from build123d import *

# Parameters (mm, degrees)
F1_DEPTH = 14
F2_R     = 5.5
F3_DEPTH = 1
F5_DEPTH = 2


with BuildPart() as f1:
    # F0 (on Top) → F1 (new body)
    with BuildSketch(Plane.XY):
        Polygon((-12.25, 0.3), (-12.25, 9), (-28.25, 9), (-28.25, -9), (12.25, -9), (12.25, 0.3), align=None)
        Polygon((28.25, -9), (28.25, 9), (12.25, 9), (12.25, 0.3), (12.25, -9), align=None)
    extrude(amount=F1_DEPTH)

    # F2 (on face) → F3 (join)
    with BuildSketch(Plane(origin=(0, 9, 0), x_dir=(-1, 0, 0), z_dir=(0, 1, 0))):
        with Locations((-20.25, 7)):
            Circle(F2_R)
        with Locations((20.25, 7)):
            Circle(F2_R)
    extrude(amount=F3_DEPTH)

    # F4 (on face) → F5 (join)
    with BuildSketch(Plane.XZ.offset(9)):
        Polygon((-6.25, 3.5), (0, 3.5), (6.25, 3.5), (6.25, 10.5), (0, 10.5), (-6.25, 10.5), align=None)
    extrude(amount=F5_DEPTH)


solid = f1.part
Model file for the job. Use its own axes, mm. A direction names the side the tool comes from. Coordinates: 2 decimals unless noted, no trailing zeros. Order: outer loops, then holes, each group sorted by start corner. A loop starts at its lowest first (then second) coordinate and runs counter-clockwise, first axis right, second up. Notation, with made-up numbers: M -11.5,-8.75 L 6.5,-8.75 A29 ccw 6.5,14.25 Z; hole C 74,35.5 d7. An arc over 180 degrees is marked long. Return JSON: item names as keys, results as strings.
1. Saw through at A-A (y = 4.5). Give the cut face in (x, z).
Ans:
{"outline": "M -28.25,0 L -12.25,0 L -12.25,14 L -28.25,14 Z; M 12.25,0 L 28.25,0 L 28.25,14 L 12.25,14 Z"}
2. Saw through at D-D (z = 3). Give the cut face in (x, y).
Ans:
{"outline": "M -28.25,-9 L 28.25,-9 L 28.25,9 L 24.02,9 L 24.02,10 L 16.48,10 L 16.48,9 L 12.25,9 L 12.25,0.3 L -12.25,0.3 L -12.25,9 L -16.48,9 L -16.48,10 L -24.02,10 L -24.02,9 L -28.25,9 Z"}
3. Tool access for faces 4 (the face through (0, -10, 10.5)), 5 (the face through (-20, 10, 7)), 6 (the face through (12.25, 5, 7)), 7 (the face through (-6.25, -10, 7)), 8 (the face through (26, 9, 8)): list every direction of +Z, -Z, +X, -X, +Y, -Y with a clear straight run to the whole face (end or side of a thin tool).
Ans:
{"face 4": "+Z, +X, -X, -Y", "face 5": "+Z, -Z, +X, -X, +Y", "face 6": "+Z, -Z, +Y", "face 7": "+Z, -Z, -X, -Y", "face 8": "+Y"}
4. Drill centre lines: probe 1 along X at (y, z) = (2.75, 2.75); probe 2 along Y at (x, z) = (-11, 5); probe 3 along Y at (x, z) = (-16.5, 6.5). Where is each one in solid material? Low to high.
Ans:
{"probe 1": "-28.25 to -12.25, 12.25 to 28.25", "probe 2": "-9 to 0.3", "probe 3": "-9 to 10"}
5. Flat gauge pins, fed straight in: pin 1 (7 mm diameter, centred on x = -12.5, z = 10, fed in from -Y); pin 2 (1.6 mm diameter, centred on y = -10, z = 8, fed in from -X); pin 3 (1 mm diameter, centred on x = 2, y = -10.5, fed in from +Z). Where does each tip first touch, or does it go through?
Ans:
{"pin 1": "y = -9", "pin 2": "x = -6.25", "pin 3": "z = 10.5"}
6. Saw through at B-B (z = 7). Give the cut face in (x, y), and give its area (3 significant figures).
Ans:
{"outline": "M -28.25,-9 L -6.25,-9 L -6.25,-11 L 6.25,-11 L 6.25,-9 L 28.25,-9 L 28.25,9 L 25.75,9 L 25.75,10 L 14.75,10 L 14.75,9 L 12.25,9 L 12.25,0.3 L -12.25,0.3 L -12.25,9 L -14.75,9 L -14.75,10 L -25.75,10 L -25.75,9 L -28.25,9 Z", "area": "851 mm^2"}
7. Saw through at C-C (x = -20.25). Give the cut face in (y, z), and give its area (3 significant figures).
Ans:
{"outline": "M -9,0 L 9,0 L 9,1.5 L 10,1.5 L 10,12.5 L 9,12.5 L 9,14 L -9,14 Z", "area": "263 mm^2"}
8. Pull direction X, two halves, no side cores. Call faces 1 (the face through (0, -10, 3.5)), 2 (the face through (6.25, -10, 7)), 3 (the face through (15.17, 9.49, 4.89)): +X half, -X half, draft (parallel to the pull), parting line (faces both ways), or undercut.
Ans:
{"face 1": "draft", "face 2": "+X half", "face 3": "undercut"}
